from build123d import *

# Parameters (mm, degrees)
F0_R      = 12
F1_DEPTH  = 104
F2_R      = 13
F3_DEPTH  = 8
F5_DEPTH  = 25
F8_DEPTH  = 79
F10_DEPTH = 10.001
F11_W     = 2
F11_H     = 5
F12_DEPTH = 6
F14_R     = 5.5
F15_DEPTH = 5.301
F16_W     = 5.875
F16_H     = 4
F17_DEPTH = 0.8
F18_R     = 1
F19_DEPTH = 20.4037756377
F21_DEPTH = 12


with BuildPart() as f1:
    # F0 (on Top) → F1 (new body)
    with BuildSketch(Plane.XY):
        Circle(F0_R)
    extrude(amount=-F1_DEPTH)

    # F2 (on face) → F3 (join)
    with BuildSketch(Plane.XY):
        Circle(F2_R)
    extrude(amount=F3_DEPTH)

    # F4 (on Top) → F5 (cut, symmetric)
    with BuildSketch(Plane.XY):
        Polygon((-4, 2), (-9.875, 2), (-9.875, -2), (9.875, -2), (9.875, 2), (4, 2), (4, 6), (-4, 6), align=None)
    extrude(amount=F5_DEPTH, both=True, mode=Mode.SUBTRACT)

    # F7 (on offset) → F8 (cut)
    with BuildSketch(Plane(origin=(0, 0, -94), x_dir=(1, 0, 0), z_dir=(0, 0, -1))):
        with BuildLine():
            Line((12.2474487139, -4.3588989435), (9, -4.3588989435))
            ThreePointArc((9, -4.3588989435), (0, 10), (-9, -4.3588989435))
            Line((-9, -4.3588989435), (-12.2474487139, -4.3588989435))
            ThreePointArc((-12.2474487139, -4.3588989435), (0, -13), (12.2474487139, -4.3588989435))
        make_face()
    extrude(amount=-F8_DEPTH, mode=Mode.SUBTRACT)

    # F9 (on offset) → F10 (cut, through all)
    with BuildSketch(Plane(origin=(0, 0, -94), x_dir=(1, 0, 0), z_dir=(0, 0, -1))):
        with BuildLine():
            Line((7.2, -7.4027756377), (-7.2, -7.4027756377))
            Line((-7.2, -7.4027756377), (-7.2, -10.8240473022))
            ThreePointArc((-7.2, -10.8240473022), (0, -13), (7.2, -10.8240473022))
            Line((7.2, -10.8240473022), (7.2, -7.4027756377))
        make_face()
    extrude(amount=F10_DEPTH, mode=Mode.SUBTRACT)

    # F11 (on face) → F12 (cut)
    with BuildSketch(Plane(origin=(0, 0, -104), x_dir=(1, 0, 0), z_dir=(0, 0, -1))):
        with Locations((0, 11.5)):
            Rectangle(F11_W, F11_H)
    extrude(amount=-F12_DEPTH, mode=Mode.SUBTRACT)

    # F14 (on offset) → F15 (cut, through all)
    with BuildSketch(Plane.XZ.offset(7.7)):
        with Locations((0, -98)):
            Circle(F14_R)
    extrude(amount=F15_DEPTH, mode=Mode.SUBTRACT)

    # F16 (on face) → F17 (join)
    with BuildSketch(Plane.XY.offset(8)):
        with Locations((-6.9375, 0)):
            Rectangle(F16_W, F16_H)
        with Locations((6.9375, 0)):
            Rectangle(F16_W, F16_H)
    extrude(amount=-F17_DEPTH)

    # F18 (on face) → F19 (cut, through all)
    with BuildSketch(Plane(origin=(0, 7.4027756377, 0), x_dir=(-1, 0, 0), z_dir=(0, 1, 0))):
        with Locations((0, -99)):
            Circle(F18_R)
    extrude(amount=-F19_DEPTH, mode=Mode.SUBTRACT)

    # F20 (on face) → F21 (cut)
    with BuildSketch(Plane.XZ.offset(7.7)):
        Polygon((0.0404706976, -101.4245333825), (2.1199428503, -100.177218039), (2.0794721527, -97.7526846565), (-0.0404706976, -96.5754666175), (-2.1199428503, -97.822781961), (-2.0794721527, -100.2473153435), align=None)
    extrude(amount=-F21_DEPTH, mode=Mode.SUBTRACT)


solid = f1.part
Geometry check sheet. Reference: the model listing, model coordinates, mm. A direction names the side the tool comes from. Round coordinates to 2 decimals unless told otherwise and drop trailing zeros. Loops run counter-clockwise (first coordinate to the right, second up) from the corner with the lowest first, then second, coordinate; pieces in that order, holes last.
Item 1: Gauge pin test, flat ends, axial feed: pin 1 (1.1 mm diameter, centred on x = -10, z = -56.5, fed in from +Y); pin 2 (1.5 mm diameter, centred on x = -10, y = 9.5, fed in from -Z); pin 3 (6 mm diameter, centred on y = -5, z = -52, fed in from +X); pin 4 (12 mm diameter, centred on x = -4.5, z = -55.5, fed in from -Y). Record the tip position at first contact, or that the pin passes through.
Item 2: Cross-section at A-A on y = 0. Record the boundary of the cut face in (x, z) (3 decimals), then the cut area to 3 significant figures.
Item 3: Cross-section at C-C on y = -6.25. Record the boundary of the cut face in (x, z).
Item 4: Cross-section at B-B on z = -99. Record the boundary of the cut face in (x, y), then the cut area to 3 significant figures.
Item 5: Access from +Z, -Z, +X, -X, +Y, -Y to the whole of each face (thin tool, end or side, straight path). Record for faces 1 (the flat face through (-7, 2, -2)), 2 (the flat face through (10, 4.359, -55)), 3 (the cylindrical face through (-2.601, -11.715, -51.272)), 4 (the flat face through (4, 5, -3)).
Item 6: Mould release check, pull along Y, two halves, no side actions. Record for faces 5 (the flat face through (1.1, -7.7, -96.6)), 6 (the cylindrical face through (-10.316, -7.91, 3.944)), 7 (the flat face through (-9.875, 0, -5)): pulls with the +Y half, pulls with the -Y half, needs draft (parallel to the pull), parting line crosses it, or undercut.
Item 7: Cross-section at D-D on z = -73. Record the boundary of the cut face in (x, y), then the cut area to 3 significant figures.
Item 8: Thickness scan on line 1 (Z direction, x = 0.75, y = -5); line 2 (X direction, y = 0, z = -64.5); line 3 (Z direction, x = 1.75, y = -5.25). Record the ranges inside material, lowest first.
Answer sheet:
1. pin 1: stops at y = 4.36
1. pin 2: passes through
1. pin 3: stops at x = 11.83
1. pin 4: stops at y = -12
2. outline: (-13, 0) - (-12, 0) - (-12, -104) - (12, -104) - (12, 0) - (13, 0) - (13, 8) - (4, 8) - (4, 7.2) - (9.875, 7.2) - (9.875, -15) - (10, -15) - (10, -94) - (-10, -94) - (-10, -15) - (-9.875, -15) - (-9.875, 7.2) - (-4, 7.2) - (-4, 8) - (-13, 8) - close; hole (-2.12, -97.823) - (-2.079, -100.247) - (0.04, -101.425) - (2.12, -100.177) - (2.079, -97.753) - (-0.04, -96.575) - close
2. area: 664 mm2
3. outline: (-11.4, 0) - (-10.24, 0) - (-10.24, -104) - (10.24, -104) - (10.24, 0) - (11.4, 0) - (11.4, 8) - (-11.4, 8) - close; hole (-7.81, -94) - (7.81, -94) - (7.81, -15) - (-7.81, -15) - close; hole (-2.12, -97.82) - (-2.08, -100.25) - (0.04, -101.42) - (2.12, -100.18) - (2.08, -97.75) - (-0.04, -96.58) - close
4. outline: (-7.2, 7.4) - (-7.2, 9.6) arc R12 ccw to (-5.41, -10.71) - (-5.41, -7.7) - (-2.1, -7.7) - (-2.1, 4.3) - (-1, 4.3) - (-1, 7.4) - close; (1, 4.3) - (2.1, 4.3) - (2.1, -7.7) - (5.41, -7.7) - (5.41, -10.71) arc R12 ccw to (7.2, 9.6) - (7.2, 7.4) - (1, 7.4) - close
4. area: 299 mm2
5. face 1: none
5. face 2: +X, -X, +Y
5. face 3: -Z
5. face 4: +Z
6. face 5: pulls with the -Y half
6. face 6: parting line crosses it
6. face 7: undercut
7. outline: (-11.18, 4.36) arc R12 ccw (long way) to (11.18, 4.36) - (9, 4.36) arc R10 cw (long way) to (-9, 4.36) - close
7. area: 87.0 mm2
8. line 1: z = -104 to -101, -97.01 to -94, -15 to 8
8. line 2: x = -12 to -10, 10 to 12
8. line 3: z = -104 to -100.4, -97.57 to -94, -15 to 8
